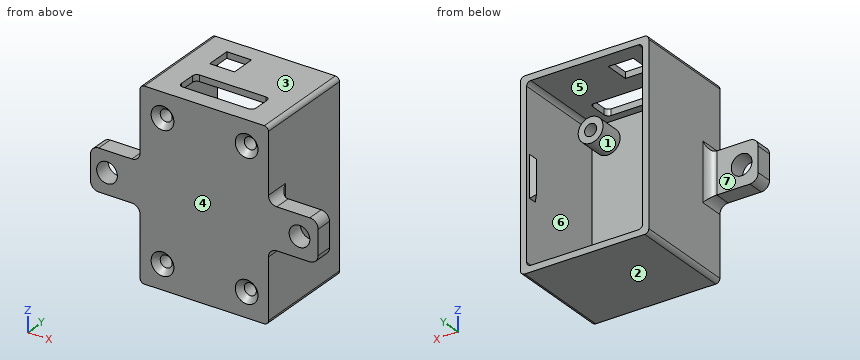
from build123d import *

# Parameters (mm, degrees)
SKETCH1_W                                         = 31
SKETCH1_H                                         = 45
BOSS_EXTRUDE1_DEPTH                               = 25
SKETCH2_W                                         = 28
SKETCH2_H                                         = 42
CUT_EXTRUDE1_DEPTH                                = 23
SKETCH3_R                                         = 3
BOSS_EXTRUDE5_DEPTH                               = 6
SKETCH4_W                                         = 18
SKETCH4_H                                         = 6
SKETCH4_W_2                                       = 6
CUT_EXTRUDE2_DEPTH                                = 1.5
CSK_FOR_M2_5_FLAT_HEAD_MACHINE_SCREW1_D           = 2.9
CSK_FOR_M2_5_FLAT_HEAD_MACHINE_SCREW1_CSINK_D     = 5.5
CSK_FOR_M2_5_FLAT_HEAD_MACHINE_SCREW1_CSINK_ANGLE = 90
FILLET2_R                                         = 1
SKETCH8_W                                         = 12
SKETCH8_H                                         = 10
BOSS_EXTRUDE6_DEPTH                               = 4
SKETCH9_R                                         = 2.5
CUT_EXTRUDE3_DEPTH                                = 4
FILLET3_R                                         = 2
FILLET4_R                                         = 2
SKETCH10_W                                        = 10
SKETCH10_H                                        = 2
BOSS_EXTRUDE7_DEPTH                               = 1
CHAMFER1_SIZE                                     = 1
SKETCH11_W                                        = 10
SKETCH11_H                                        = 2
BOSS_EXTRUDE8_DEPTH                               = 1
CHAMFER2_SIZE                                     = 1
FILLET5_R                                         = 2


with BuildPart() as part:
    # Sketch1 → Boss-Extrude1 (new body)
    with BuildSketch(Plane(origin=(0, 0, 0), x_dir=(1, 0, 0), z_dir=(0, 1, 0))):
        Rectangle(SKETCH1_W, SKETCH1_H)
    extrude(amount=BOSS_EXTRUDE1_DEPTH)

    # Sketch2 → Cut-Extrude1 (cut)
    with BuildSketch(Plane(origin=(0, 25, 0), x_dir=(1, 0, 0), z_dir=(0, 1, 0))):
        Rectangle(SKETCH2_W, SKETCH2_H)
    extrude(amount=-CUT_EXTRUDE1_DEPTH, mode=Mode.SUBTRACT)

    # Sketch3 → Boss-Extrude5 (add)
    with BuildSketch(Plane(origin=(0, 2, 0), x_dir=(1, 0, 0), z_dir=(0, 1, 0))):
        with Locations(Location((-10.090049644, 16.575, 0), (0, 0, 270))):
            Circle(SKETCH3_R)
        with Locations(Location((10.229950356, 16.575, 0), (0, 0, 270))):
            Circle(SKETCH3_R)
        with Locations(Location((10.229950356, -16.575, 0), (0, 0, 270))):
            Circle(SKETCH3_R)
        with Locations(Location((-10.090049644, -16.575, 0), (0, 0, 270))):
            Circle(SKETCH3_R)
    extrude(amount=BOSS_EXTRUDE5_DEPTH)

    # Sketch4 → Cut-Extrude2 (cut)
    with BuildSketch(Plane.XY.offset(22.5)):
        with Locations((0, 7)):
            Rectangle(SKETCH4_W, SKETCH4_H)
        with Locations((-6, 18)):
            Rectangle(SKETCH4_W_2, SKETCH4_H)
    extrude(amount=-CUT_EXTRUDE2_DEPTH, mode=Mode.SUBTRACT)

    # CSK for M2.5 Flat Head Machine Screw1 (through all)
    with Locations(Plane(origin=(0, 0, 0), x_dir=(-1, 0, 0), z_dir=(0, -1, 0))):
        with Locations((-10.229950356, -16.575), (10.090049644, -16.575), (10.090049644, 16.575), (-10.229950356, 16.575)):
            CounterSinkHole(CSK_FOR_M2_5_FLAT_HEAD_MACHINE_SCREW1_D / 2, CSK_FOR_M2_5_FLAT_HEAD_MACHINE_SCREW1_CSINK_D / 2, counter_sink_angle=CSK_FOR_M2_5_FLAT_HEAD_MACHINE_SCREW1_CSINK_ANGLE)

    # Fillet2
    fillet2_edges = [part.edges().sort_by_distance(p)[0] for p in [
        (14, 13.5, -21),
        (14, 13.5, 21),
        (-14, 13.5, 21),
        (-14, 13.5, -21),
        (-9, 4, 21.75),
        (-9, 10, 21.75),
        (9, 10, 21.75),
        (9, 4, 21.75),
        (15.5, 12.5, 22.5),
        (-15.5, 12.5, 22.5),
        (-15.5, 12.5, -22.5),
        (15.5, 12.5, -22.5),
    ]]
    fillet(fillet2_edges, radius=FILLET2_R)

    # Sketch8 → Boss-Extrude6 (add)
    with BuildSketch(Plane(origin=(0, 0, 0), x_dir=(1, 0, 0), z_dir=(0, 1, 0))):
        with Locations((21.5, 0)):
            Rectangle(SKETCH8_W, SKETCH8_H)
        with Locations((-21.5, 0)):
            Rectangle(SKETCH8_W, SKETCH8_H)
    extrude(amount=BOSS_EXTRUDE6_DEPTH)

    # Sketch9 → Cut-Extrude3 (cut)
    with BuildSketch(Plane(origin=(0, 4, 0), x_dir=(1, 0, 0), z_dir=(0, 1, 0))):
        with Locations(Location((23, 0, 0), (0, 0, 270))):
            Circle(SKETCH9_R)
        with Locations(Location((-23.5, 0, 0), (0, 0, 270))):
            Circle(SKETCH9_R)
    extrude(amount=-CUT_EXTRUDE3_DEPTH, mode=Mode.SUBTRACT)

    # Fillet3
    fillet3_edges = [part.edges().sort_by_distance(p)[0] for p in [
        (-15.5, 2, 5),
        (-15.5, 2, -5),
        (15.5, 2, -5),
        (15.5, 2, 5),
    ]]
    fillet(fillet3_edges, radius=FILLET3_R)

    # Fillet4
    fillet4_edges = [part.edges().sort_by_distance(p)[0] for p in [
        (15.5, 4, 0),
        (-15.5, 4, 0),
    ]]
    fillet(fillet4_edges, radius=FILLET4_R)

    # Sketch10 → Boss-Extrude7 (add)
    with BuildSketch(Plane(origin=(-14, 0, 0), x_dir=(0, 0, -1), z_dir=(1, 0, 0))):
        with Locations((0, 23)):
            Rectangle(SKETCH10_W, SKETCH10_H)
    extrude(amount=BOSS_EXTRUDE7_DEPTH)

    # Chamfer1
    chamfer1_edges = [part.edges().sort_by_distance(p)[0] for p in [
        (-13, 23, 5),
        (-13, 22, 0),
        (-13, 23, -5),
        (-13, 24, 0),
    ]]
    chamfer(chamfer1_edges, length=CHAMFER1_SIZE - 0.0001)  # a hair under: the kernel refuses the full size

    # Sketch11 → Boss-Extrude8 (add)
    with BuildSketch(Plane.ZY.offset(-14)):
        with Locations((0, 23)):
            Rectangle(SKETCH11_W, SKETCH11_H)
    extrude(amount=BOSS_EXTRUDE8_DEPTH)

    # Chamfer2
    chamfer2_edges = [part.edges().sort_by_distance(p)[0] for p in [
        (13, 23, 5),
        (13, 24, 0),
        (13, 22, 0),
        (13, 23, -5),
    ]]
    chamfer(chamfer2_edges, length=CHAMFER2_SIZE - 0.0001)  # a hair under: the kernel refuses the full size

    # Fillet5
    fillet5_edges = [part.edges().sort_by_distance(p)[0] for p in [
        (-27.5, 2, -5),
        (-27.5, 2, 5),
        (27.5, 2, 5),
        (27.5, 2, -5),
    ]]
    fillet(fillet5_edges, radius=FILLET5_R)


solid = part.part
Geometry check sheet. Reference: the model listing, model coordinates, mm. Face numbers are marked on the shaded views. A direction names the side the tool comes from. Give positions to 0.01 mm unless a question says otherwise; leave off trailing zeros. Order: outer loops, then holes, each group sorted by start corner. A loop starts at its lowest first (then second) coordinate and runs counter-clockwise, first axis right, second up.
1. Sectioned sample at A-A (x = -23.5). Record the boundary of the cut face in (y, z).
Completed:
outline: (0, -5) - (4, -5) - (4, -2.5) - (0, -2.5) - close; (0, 2.5) - (4, 2.5) - (4, 5) - (0, 5) - close
2. Sectioned sample at D-D (y = 18.25). Record the boundary of the cut face in (x, z).
Completed:
outline: (-15.5, -21.5) arc R1 ccw to (-14.5, -22.5) - (14.5, -22.5) arc R1 ccw to (15.5, -21.5) - (15.5, 21.5) arc R1 ccw to (14.5, 22.5) - (-3, 22.5) - (-3, 21) - (13, 21) arc R1 cw to (14, 20) - (14, -20) arc R1 cw to (13, -21) - (-13, -21) arc R1 cw to (-14, -20) - (-14, 20) arc R1 cw to (-13, 21) - (-9, 21) - (-9, 22.5) - (-14.5, 22.5) arc R1 ccw to (-15.5, 21.5) - close
3. Access from +Z, -Z, +X, -X, +Y, -Y to the whole of each face (thin tool, end or side, straight path). Record for the marked faces 5, 6 and 7.
Completed:
face 5: +Y
face 6: none
face 7: +Z, -Z, -X, +Y
4. Sectioned sample at C-C (y = 11). Record the boundary of the cut face in (x, z).
Completed:
outline: (-15.5, -21.5) arc R1 ccw to (-14.5, -22.5) - (14.5, -22.5) arc R1 ccw to (15.5, -21.5) - (15.5, 21.5) arc R1 ccw to (14.5, 22.5) - (-14.5, 22.5) arc R1 ccw to (-15.5, 21.5) - close; hole (-14, -20) arc R1 ccw to (-13, -21) - (13, -21) arc R1 ccw to (14, -20) - (14, 20) arc R1 ccw to (13, 21) - (-13, 21) arc R1 ccw to (-14, 20) - close
5. Scan lines: line 1 (X direction, y = 2.7, z = 0); line 2 (X direction, y = 17, z = -3.5); line 3 (Z direction, x = -8.5, y = 3). Record each from-to range of solid material in increasing order.
Completed:
line 1: x = -27.5 to -26, -21 to -14, 14 to 20.5, 25.5 to 27.5
line 2: x = -15.5 to -14, 14 to 15.5
line 3: z = -22.5 to -21, -19.12 to -14.03, 14.03 to 19.12, 21 to 22.5
6. Sectioned sample at B-B (z = 0). State how many separate pieces and enclosed holes the cut face has, then the cut area to 3 significant figures.
Completed:
separate pieces: 3
enclosed holes: 0
area: 191 mm2
7. Depth check by flat-ended pin: pin 1 (10 mm diameter, centred on x = 1.5, z = -2, fed in from +Y); pin 2 (3 mm diameter, centred on y = 4.5, z = -14.5, fed in from -X); pin 3 (3 mm diameter, centred on x = 20.5, y = 1.5, fed in from -Z). Enter the tip coordinate at first touch or a pass-through.
Completed:
pin 1: stops at y = 2
pin 2: stops at x = -15.5
pin 3: stops at z = -5
8. Draft check along Z on the marked faces 1, 2, 3 and 4. Enter one of: pulls with the +Z half, pulls with the -Z half, needs draft (parallel to the pull), parting line crosses it, or undercut.
Completed:
face 1: undercut
face 2: pulls with the -Z half
face 3: pulls with the +Z half
face 4: needs draft
